Autodesk Fusion 360 part; units mm, degrees
sketch "Sketch1" plane through (0, 0, 0) normal (0, 0, 1) x (1, 0, 0)
  line L0 (0, 0) -> (14, 0)
  line L1 (14, 0) -> (14, 14)
  line L2 (14, 14) -> (0, 14)
  line L3 (0, 14) -> (0, 0)
  line L4 (0, 12.4) -> (14, 12.4)
  line L5 (0, 1.6) -> (14, 1.6)
  dimension "d1" = 14
  dimension "d2" = 14
  dimension "d3" = 1.6
  dimension "d4" = 1.6
extrude "Extrude1" add sketch "Sketch1" along normal blind 1.4
extrude "Extrude2" add sketch "Sketch1" along normal blind 4 contours L0 L1 L3 L5 | L1 L2 L3 L4
For this review, take the finished solid that the model builds, in its own axes (mm). A direction names the side the tool comes from. Coordinates: 2 decimals unless noted, no trailing zeros. Write each loop counter-clockwise with the first axis right and the second up, starting at its lowest first coordinate (ties: lowest second). Pieces come first, ordered by that corner, then holes. Notation, with made-up numbers: (32, 17) - (68, 17) arc R34 cw to (68, 53) - close; hole circle Ø9 at (-38, 22). An arc over 180 degrees is marked (long way). Answer in a Markdown table with one row per item. Add a question column.
Q1. We need section A-A, the plane z = 2.8. State the section outline as (x, y) points.
Q2. Draft analysis for pull direction Y (two halves, no side actions). For faces 1 (the flat face through (7, 0, 2)), 2 (the flat face through (7, 7, 1.4)), 3 (the flat face through (7, 1.6, 3)), 4 (the flat face through (7, 13, 4)), state which applies: +Y half, -Y half, draft (parallel to the pull), parting line (faces both ways), or undercut.
Q3. For P1, Ø2, axis at x = 8.5, z = 3.5, coming from the -Y side; P2, Ø2, axis at y = 7.5, z = 3.5, coming from the -X side; P3, Ø4, axis at x = 2, y = 7, coming from the +Z side, all flat-tipped, find the tip position at first contact; note any pin that passes through.
Q4. For probe 1 along Y at (x, z) = (2.25, 3.5); probe 2 along Z at (x, y) = (1, 7.5), list the stretches that pass through material, from the lowest coordinate up.
Q5. We need section C-C, the plane y = 3. State the section outline as (x, z) points, and give its area (3 significant figures).
Q6. Tool access review of faces 5 (the flat face through (7, 12.4, 3)), 6 (the flat face through (14, 7, 1)): name each direction out of +Z, -Z, +X, -X, +Y, -Y from which nothing blocks a thin tool from reaching the whole face with its end or side.
Q7. We need section B-B, the plane x = 12.5. State the section outline as (y, z) points.
Answer list:
| question | item | result |
|---|---|---|
| 1 | outline | (0, 0) - (14, 0) - (14, 1.6) - (0, 1.6) - close; (0, 12.4) - (14, 12.4) - (14, 14) - (0, 14) - close |
| 2 | face 1 | -Y half |
| 2 | face 2 | undercut |
| 2 | face 3 | undercut |
| 2 | face 4 | draft |
| 3 | P1 | stops at y = 0 |
| 3 | P2 | passes through |
| 3 | P3 | stops at z = 1.4 |
| 4 | probe 1 | y = 0 to 1.6, 12.4 to 14 |
| 4 | probe 2 | z = 0 to 1.4 |
| 5 | outline | (0, 0) - (14, 0) - (14, 1.4) - (0, 1.4) - close |
| 5 | area | 19.6 mm2 |
| 6 | face 5 | +Z, +X, -X |
| 6 | face 6 | +Z, -Z, +X, +Y, -Y |
| 7 | outline | (0, 0) - (14, 0) - (14, 4) - (12.4, 4) - (12.4, 1.4) - (1.6, 1.4) - (1.6, 4) - (0, 4) - close |
